For this review, take the finished solid that the model builds, in its own axes (mm). A direction names the side the tool comes from. Coordinates: 2 decimals unless noted, no trailing zeros.
from build123d import *

# Parameters (mm, degrees)
CUT_EXTRUDE1_DEPTH = 22.708736000744032


with BuildPart() as part:
    # Sketch1 → Revolve1 (revolve)
    with BuildSketch(Plane.XY, mode=Mode.PRIVATE) as revolve1_sk:
        Polygon((0.254, 14.2875), (7.6835, 14.2875), (7.9375, 14.033499999999998), (7.9375, 12.7), (7.556499999999999, 12.7), (7.5565, 10.16), (7.9375, 10.16), (7.9375, 7.9374999999999964), (6.349999999999997, 6.349999999999998), (1.587500000000001, 6.3500000000000005), (0, 7.9375), (0, 10.16), (0.381, 10.16), (0.381, 12.7), (0, 12.7), (0, 14.033499999999998), align=None)
    revolve(revolve1_sk.sketch.rotate(Axis((0, 0, 0), (-1, 0, 0)), 90), axis=Axis((0, 0, 0), (-1, 0, 0)))

    # Sketch2 → Cut-Extrude1 (cut, through all)
    with BuildSketch(Plane(origin=(7.9375, 0, 0), x_dir=(0, 0, -1), z_dir=(1, 0, 0))):
        Polygon((-8.7e-16, 7.332348418708245), (-6.349999999999997, 3.6661742093541227), (-6.349999999999996, -3.666174209354121), (5.15e-15, -7.332348418708244), (6.349999999999999, -3.6661742093541214), (6.349999999999997, 3.6661742093541236), align=None)
    extrude(amount=-CUT_EXTRUDE1_DEPTH, mode=Mode.SUBTRACT)


solid = part.part
1. To check wall thickness, follow L1, parallel to Y at x = 7.85, z = 0; L2, parallel to Y at x = 0.3, z = 0; L3, parallel to Y at x = 1.75, z = 4.75. State the ranges of each line that lie inside material, in increasing order.
Answer below:
L1: y = -14.12 to -12.7, -10.16 to -7.85, 7.85 to 10.16, 12.7 to 14.12
L2: y = -14.29 to -12.7, -10.16 to -7.64, 7.64 to 10.16, 12.7 to 14.29
L3: y = -13.47 to -4.59, 4.59 to 13.47
2. The part is to be moulded in two halves that separate along Z. For faces 1 (the face through (0, 2, -13)), 2 (the face through (4.016, -5.525, -3.131)), 3 (the face through (4, 0, 6.35)), say which applies: +Z half, -Z half, draft (parallel to the pull), parting line (faces both ways), or undercut.
Answer below:
face 1: draft
face 2: undercut
face 3: undercut
3. Machinability: for faces 4 (the face through (4.016, -5.474, 3.219)), 5 (the face through (0.2, 7.7, 10.1)), 6 (the face through (0, 4.5, -6.8)), 7 (the face through (7.744, 7.728, 10.078)), which of the approach directions +Z, -Z, +X, -X, +Y, -Y give a long, thin tool a straight path to every point of the face, cutting with its end or side? Answer none if there is none.
Answer below:
face 4: +X, -X
face 5: -X
face 6: +Z, -Z, -X, +Y, -Y
face 7: +X
4. Clearance check with flat-ended pins moving along their axes: pin 1 Ø6 at (y, z) = (3, -2.5) entering from -X; pin 2 Ø4 at (x, y) = (1, -5.5) entering from +Z; pin 3 Ø3 at (y, z) = (-3, -5) entering from +X; pin 4 Ø5 at (y, z) = (0, 1.5) entering from +X. State where each tip first meets the part, or that it passes through.
Answer below:
pin 1: stops at x = 1.03
pin 2: stops at z = 13.85
pin 3: stops at x = 7.33
pin 4: passes through
